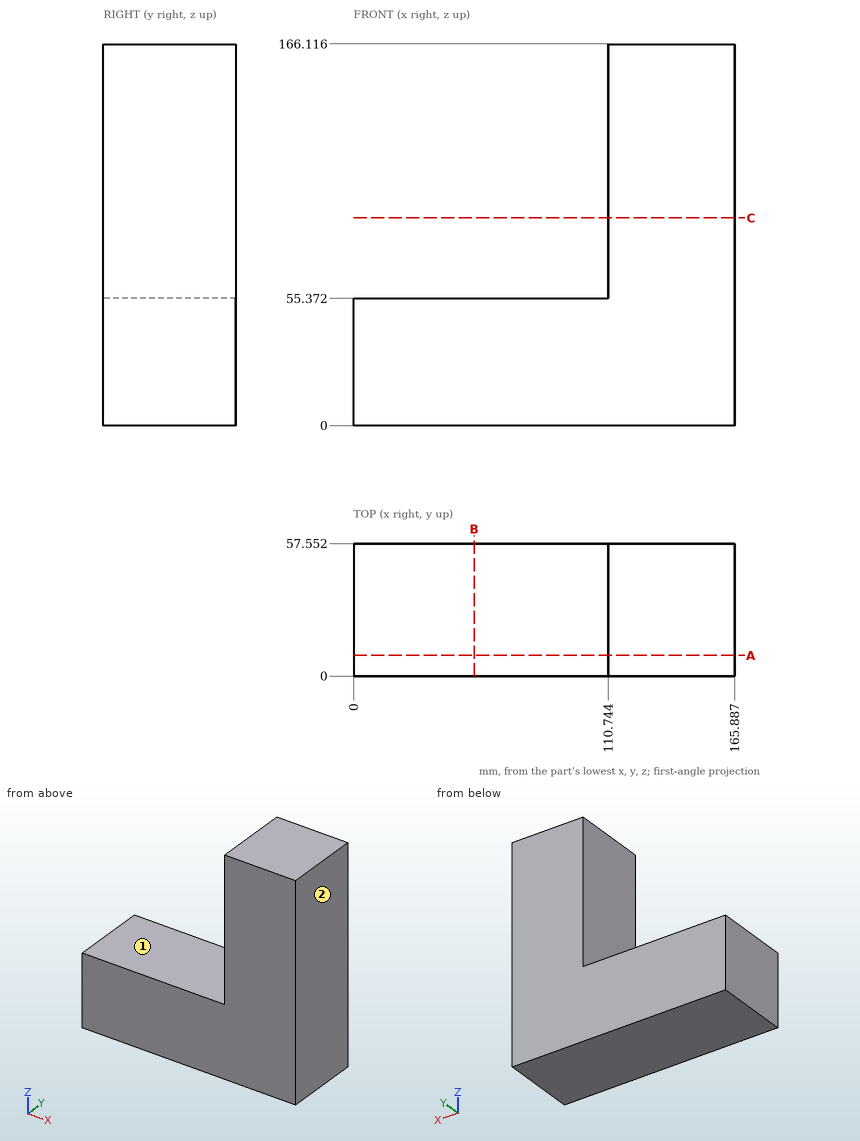
Print and shaded views of the part. All mm, measured from the part's lowest x, y and z. A direction names the side the tool comes from. Give positions to 0.01 mm unless a question says otherwise; leave off trailing zeros. Order: outer loops, then holes, each group sorted by start corner. A loop starts at its lowest first (then second) coordinate and runs counter-clockwise, first axis right, second up. Notation, with made-up numbers: (74, 19) - (110, 19) arc R13 cw to (110, 40) - close; hole circle Ø5 at (60.5, -18.5). An arc over 180 degrees is marked (long way). Use a Markdown table: item, result.
1) Saw through at C-C on z = 90.5. List the corners of the cut face in (x, y), plus the area to 3 significant figures.
Checked values:
| item | result |
|---|---|
| outline | (110.74, 0) - (165.89, 0) - (165.89, 57.55) - (110.74, 57.55) - close |
| area | 3,170 mm² |
2) Flat gauge pins, fed straight in: P1, Ø17.5, axis at x = 71.5, y = 30, coming from the +Z side; P2, Ø1, axis at y = 26, z = 118.5, coming from the -X side. Where does each tip first touch, or does it go through?
Checked values:
| item | result |
|---|---|
| P1 | z = 55.37 |
| P2 | x = 110.74 |
3) 3-axis set-ups, long thin cutter, end or side, ignore diameter. For the marked faces 1 and 2: which of +Z, -Z, +X, -X, +Y, -Y reach the whole face in a straight line?
Checked values:
| item | result |
|---|---|
| face 1 | +Z, -X, +Y, -Y |
| face 2 | +Z, -Z, +X, +Y, -Y |
4) Saw through at B-B on x = 52.5. List the corners of the cut face in (y, z).
Checked values:
| item | result |
|---|---|
| outline | (0, 0) - (57.55, 0) - (57.55, 55.37) - (0, 55.37) - close |
5) Saw through at A-A on y = 9. List the corners of the cut face in (x, z), plus the area to 3 significant figures.
Checked values:
| item | result |
|---|---|
| outline | (0, 0) - (165.89, 0) - (165.89, 166.12) - (110.74, 166.12) - (110.74, 55.37) - (0, 55.37) - close |
| area | 15,300 mm² |
6) Probe L1, parallel to X at y = 14.5, z = 141; L2, parallel to Z at x = 51, y = 36. List the from-to ranges inside material, lowest first. Write a range as from..to.
Checked values:
| item | result |
|---|---|
| L1 | 110.74..165.89 |
| L2 | 0..55.37 |
